For this review, take the finished solid that the model builds, in its own axes (mm). A direction names the side the tool comes from. Give positions to 0.01 mm unless a question says otherwise; leave off trailing zeros. Order: outer loops, then holes, each group sorted by start corner. A loop starts at its lowest first (then second) coordinate and runs counter-clockwise, first axis right, second up.
from build123d import *

# Parameters (mm, degrees)
SKETCH_1_R               = 18.25
EXTRUDE_1_DEPTH          = 25
SKETCH_2_R               = 12.5
CUT_EXTRUDE_1_DEPTH      = 25
SKETCH_3_W               = 120
SKETCH_3_H               = 40
EXTRUDE_2_DEPTH          = 65
SKETCH_5_W               = 20
SKETCH_5_H               = 55
CUT_EXTRUDE_2_DEPTH      = 30
SKETCH_6_W               = 20
SKETCH_6_H               = 40
CUT_EXTRUDE_3_DEPTH      = 30
SKETCH_7_W               = 4
SKETCH_7_H               = 55
CUT_EXTRUDE_4_DEPTH      = 5
SKETCH_8_R               = 5
EXTRUDE_4_DEPTH          = 12
CUT_EXTRUDE_5_DEPTH      = 113.800709218
CUT_EXTRUDE_5_DEPTH_BACK = 60
SKETCH_9_W               = 120
SKETCH_9_H               = 16
SKETCH_10_W              = 40
SKETCH_10_H              = 25
EXTRUDE_5_DEPTH          = 13.5
SKETCH_13_R              = 2
CUT_EXTRUDE_6_DEPTH      = 30
SKETCH_14_R              = 15
EXTRUDE_6_DEPTH          = 6.5
EXTRUDE_START            = 6.5
SKETCH_15_W              = 40
SKETCH_15_H              = 12
SKETCH_15_R              = 2
EXTRUDE_7_DEPTH          = 6.5
FILLET_1_R               = 10
FILLET_2_R               = 10
FILLET_3_R               = 1
CHAMFER_1_SIZE           = 0.5


with BuildPart() as part:
    # 草图1 → 凸台-拉伸1 (new body)
    with BuildSketch(Plane.XY):
        Circle(SKETCH_1_R)
    extrude(amount=EXTRUDE_1_DEPTH)

    # 草图2 → 切除-拉伸1 (cut)
    with BuildSketch(Plane.XY.offset(25)):
        Circle(SKETCH_2_R)
    extrude(amount=-CUT_EXTRUDE_1_DEPTH, mode=Mode.SUBTRACT)

    # 草图3 → 凸台-拉伸2 (add)
    with BuildSketch(Plane.XY.offset(25)):
        Rectangle(SKETCH_3_W, SKETCH_3_H)
    extrude(amount=EXTRUDE_2_DEPTH)

    # 草图5 → 切除-拉伸2 (cut)
    with BuildSketch(Plane.XZ.offset(20)):
        with Locations((28, 57.5)):
            Rectangle(SKETCH_5_W, SKETCH_5_H)
    extrude(amount=-CUT_EXTRUDE_2_DEPTH, mode=Mode.SUBTRACT)

    # 草图6 → 切除-拉伸3 (cut)
    with BuildSketch(Plane.XZ.offset(-10)):
        with Locations((28, 57.5)):
            Rectangle(SKETCH_6_W, SKETCH_6_H)
    extrude(amount=-CUT_EXTRUDE_3_DEPTH, mode=Mode.SUBTRACT)

    # 草图7 → 切除-拉伸4 (cut)
    with BuildSketch(Plane.XZ.offset(-10)):
        with Locations((28, 57.5)):
            Rectangle(SKETCH_7_W, SKETCH_7_H)
    extrude(amount=-CUT_EXTRUDE_4_DEPTH, mode=Mode.SUBTRACT)

    # 草图8 → 凸台-拉伸4 (add)
    with BuildSketch(Plane(origin=(0, 20, 0), x_dir=(1, 0, 0), z_dir=(0, 1, 0))):
        with Locations(Location((-28, -67.5, 0), (0, 0, 90))):
            Circle(SKETCH_8_R)
    extrude(amount=EXTRUDE_4_DEPTH)

    # 草图9 → 切除-拉伸5 (cut, two sides: drawn at the far end of the back side and taken through both)
    with BuildSketch(Plane.XY.offset(90).offset(-CUT_EXTRUDE_5_DEPTH_BACK)):
        with Locations((0, -12)):
            Rectangle(SKETCH_9_W, SKETCH_9_H)
    extrude(amount=CUT_EXTRUDE_5_DEPTH + CUT_EXTRUDE_5_DEPTH_BACK, mode=Mode.SUBTRACT)

    # 草图10 → 凸台-拉伸5 (add)
    with BuildSketch(Plane(origin=(0, 20, 0), x_dir=(1, 0, 0), z_dir=(0, 1, 0))):
        with Locations((0, -102.5)):
            Rectangle(SKETCH_10_W, SKETCH_10_H)
    extrude(amount=-EXTRUDE_5_DEPTH)

    # 草图13 → 切除-拉伸6 (cut)
    with BuildSketch(Plane(origin=(0, 20, 0), x_dir=(1, 0, 0), z_dir=(0, 1, 0))):
        with Locations(Location((-10.600287359, -109, 0), (0, 0, 270))):
            Circle(SKETCH_13_R)
        with Locations(Location((10.600287359, -109, 0), (0, 0, 270))):
            Circle(SKETCH_13_R)
    extrude(amount=-CUT_EXTRUDE_6_DEPTH, mode=Mode.SUBTRACT)

    # 草图14 → 凸台-拉伸6 (add)
    with BuildSketch(Plane(origin=(0, 20, 0), x_dir=(1, 0, 0), z_dir=(0, 1, 0))):
        with Locations(Location((-28, -67.5, 0), (0, 0, 90))):
            Circle(SKETCH_14_R)
    extrude(amount=EXTRUDE_6_DEPTH)

    # 草图15 → 凸台-拉伸7 (add)
    with BuildSketch(Plane(origin=(0, 20, 0), x_dir=(1, 0, 0), z_dir=(0, 1, 0)).offset(EXTRUDE_START)):
        with Locations((0, -109)):
            Rectangle(SKETCH_15_W, SKETCH_15_H)
        with Locations(Location((-10.600287359, -109, 0), (0, 0, 270))):
            Circle(SKETCH_15_R, mode=Mode.SUBTRACT)
        with Locations(Location((10.600287359, -109, 0), (0, 0, 270))):
            Circle(SKETCH_15_R, mode=Mode.SUBTRACT)
    extrude(amount=-EXTRUDE_7_DEPTH)

    # 圆角1
    fillet_1_edges = [part.edges().sort_by_distance(p)[0] for p in [
        (-20, 16.5, 115),
        (20, 16.5, 115),
    ]]
    fillet(fillet_1_edges, radius=FILLET_1_R)

    # 圆角2
    fillet_2_edges = [part.edges().sort_by_distance(p)[0] for p in [
        (60, 8, 90),
        (-60, 8, 90),
    ]]
    fillet(fillet_2_edges, radius=FILLET_2_R)

    # 圆角3
    fillet_3_edges = [part.edges().sort_by_distance(p)[0] for p in [
        (0, -20, 25),
        (0, -20, 30),
    ]]
    fillet(fillet_3_edges, radius=FILLET_3_R)

    # 倒角1
    chamfer_1_edges = [part.edges().sort_by_distance(p)[0] for p in [
        (-28, 32, 72.5),
    ]]
    chamfer(chamfer_1_edges, length=CHAMFER_1_SIZE)


solid = part.part
1) We need section D-D on x = 0. Give the boundary of the cut face in (y, z), then the cut area to 3 significant figures.
Answer sheet:
outline: (-20, 26) arc R1 ccw to (-19, 25) - (-18.25, 25) - (-18.25, 0) - (-12.5, 0) - (-12.5, 25) - (12.5, 25) - (12.5, 0) - (18.25, 0) - (18.25, 25) - (20, 25) - (20, 103) - (26.5, 103) - (26.5, 115) - (6.5, 115) - (6.5, 90) - (-4, 90) - (-4, 30) - (-19, 30) arc R1 ccw to (-20, 29) - close
area: 2,340 mm2
2) Clearance check with flat-ended pins moving along their axes: pin 1 (2 mm diameter, centred on x = -45, z = 45.5, fed in from -Y); pin 2 (12 mm diameter, centred on y = 12, z = 94.5, fed in from -X); pin 3 (4.5 mm diameter, centred on x = 10.6, z = 109, fed in from -Y); pin 4 (12 mm diameter, centred on y = -8, z = 31, fed in from +X). State where each tip first meets the part, or that it passes through.
Answer sheet:
pin 1: stops at y = -4
pin 2: stops at x = -55.27
pin 3: stops at y = 6.5
pin 4: stops at x = 60
3) Draft analysis for pull direction Z (two halves, no side actions). For faces 6 (the face through (-60, 9, 52)), 7 (the face through (34, 10, 81)), 8 (the face through (-14, 14, 25)), 9 (the face through (0, 17, 115)), state which applies: +Z half, -Z half, draft (parallel to the pull), parting line (faces both ways), or undercut.
Answer sheet:
face 6: draft
face 7: undercut
face 8: -Z half
face 9: +Z half
4) To check wall thickness, follow line 1 (X direction, y = 7, z = 70.5); line 2 (Z direction, x = 10.5, y = 22.5); line 3 (X direction, y = 15, z = 109). State the ranges of each line that lie inside material, in increasing order.
Answer sheet:
line 1: x = -60 to 18, 38 to 60
line 2: z = 103 to 107, 111 to 114.99
line 3: x = -19.17 to -12.6, -8.6 to 8.6, 12.6 to 19.17
5) We need section C-C on z = 109. Give the boundary of the cut face in (x, y), then the cut area to 3 significant figures.
Answer sheet:
outline: (-19.17, 6.5) - (-12.6, 6.5) - (-12.6, 26.5) - (-19.17, 26.5) - close; (-8.6, 6.5) - (8.6, 6.5) - (8.6, 26.5) - (-8.6, 26.5) - close; (12.6, 6.5) - (19.17, 6.5) - (19.17, 26.5) - (12.6, 26.5) - close
area: 607 mm2
6) Tool access review of faces 1 (the face through (0, 26.5, 109)), 2 (the face through (0, 6.5, 102)), 3 (the face through (0, 23, 103)), 4 (the face through (28, 3, 85)), 5 (the face through (-56.99, 8.17, 87.15)): name each direction out of +Z, -Z, +X, -X, +Y, -Y from which nothing blocks a thin tool from reaching the whole face with its end or side.
Answer sheet:
face 1: +Z, -Z, +X, -X, +Y
face 2: +Z, +X, -X, -Y
face 3: +X, -X, +Y
face 4: -Y
face 5: +Z, -X, +Y, -Y
7) We need section A-A on z = 47. Give the boundary of the cut face in (x, y).
Answer sheet:
outline: (-60, -4) - (18, -4) - (18, 20) - (-60, 20) - close; (38, -4) - (60, -4) - (60, 20) - (38, 20) - close
8) We need section B-B on y = 0. Give the boundary of the cut face in (x, z), then the cut area to 3 significant figures.
Answer sheet:
outline: (-60, 25) - (-18.25, 25) - (-18.25, 0) - (-12.5, 0) - (-12.5, 25) - (12.5, 25) - (12.5, 0) - (18.25, 0) - (18.25, 25) - (60, 25) - (60, 80) arc R10 ccw to (50, 90) - (-50, 90) arc R10 ccw to (-60, 80) - close; hole (18, 30) - (38, 30) - (38, 85) - (18, 85) - close
area: 6,940 mm2
